```python
from build123d import *

# Parameters (mm, degrees)
SKETCH2_R          = 50
CUT_EXTRUDE1_DEPTH = 10
SKETCH3_R          = 1
CUT_EXTRUDE2_DEPTH = 180
SKETCH4_R          = 1
CUT_EXTRUDE3_DEPTH = 1
SKETCH5_R          = 99.5
CUT_EXTRUDE7_DEPTH = 26


with BuildPart() as part:
    # Sketch1 → Revolve1 (revolve)
    with BuildSketch(Plane.XY):
        Polygon((0, 0), (50, 0), (200, 50), (200, 101), (0, 101), align=None)
        Polygon((49.83772234, 1), (199, 50.72075922), (199, 100), (1, 100), (1, 1), align=None, mode=Mode.SUBTRACT)
    revolve(axis=Axis((0, 101, 0), (1, 0, 0)))

    # Sketch2 → Cut-Extrude1 (cut)
    with BuildSketch(Plane(origin=(200, 0, 0), x_dir=(0, 0, -1), z_dir=(1, 0, 0))):
        with Locations((0, 101)):
            Circle(SKETCH2_R)
    extrude(amount=-CUT_EXTRUDE1_DEPTH, mode=Mode.SUBTRACT)

    # Sketch3 → Cut-Extrude2 (cut)
    with BuildSketch(Plane(origin=(190, 0, 0), x_dir=(0, 0, -1), z_dir=(1, 0, 0))):
        with Locations((0, 101)):
            Circle(SKETCH3_R)
    extrude(amount=-CUT_EXTRUDE2_DEPTH, mode=Mode.SUBTRACT)

    # Sketch4 → Cut-Extrude3 (cut)
    with BuildSketch(Plane(origin=(10, 0, 0), x_dir=(0, 0, -1), z_dir=(1, 0, 0))):
        with Locations((0, 101)):
            Circle(SKETCH4_R)
    extrude(amount=-CUT_EXTRUDE3_DEPTH, mode=Mode.SUBTRACT)

    # Sketch5 → Cut-Extrude7 (cut)
    with BuildSketch(Plane.ZY):
        with Locations((0, 101)):
            Circle(SKETCH5_R)
    extrude(amount=-CUT_EXTRUDE7_DEPTH, mode=Mode.SUBTRACT)


solid = part.part
```
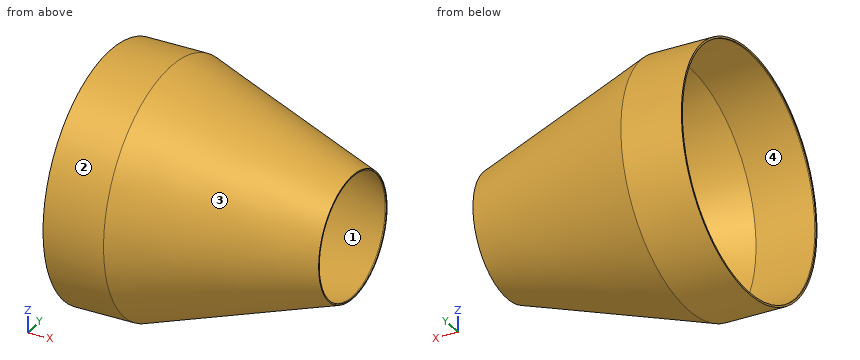
Build history of the part. All positions in model axes, mm. Face numbers are marked on the shaded views. A direction names the side the tool comes from. Give positions to 0.01 mm unless a question says otherwise; leave off trailing zeros. Loops run counter-clockwise (first coordinate to the right, second up) from the corner with the lowest first, then second, coordinate; pieces in that order, holes last.
1) 3-axis set-ups, long thin cutter, end or side, ignore diameter. For the marked faces 3 and 4: which of +Z, -Z, +X, -X, +Y, -Y reach the whole face in a straight line?
Values follow:
face 3: +X
face 4: none
2) Band-saw the part on C-C on x = 33. List the corners of the cut face in (y, z).
Values follow:
outline: circle Ø202 at (101, 0); hole circle Ø200 at (101, 0)
3) Drop flat-ended pins along their axis: P1, Ø4, axis at x = 120.5, y = 161, coming from the -Z side; P2, Ø1.5, axis at x = 159.5, y = 127.5, coming from the -Z side; P3, Ø1.5, axis at x = 165.5, z = 26, coming from the +Y side. Give the stop position or say it passes through.
Values follow:
P1: stops at z = -51.62
P2: stops at z = -59.24
P3: stops at y = 158.27
4) Two-plate mould, pull along Z, no slides. Class the marked faces 1 and 2: released by +Z, released by -Z, zero draft, split by the parting line, or undercut.
Values follow:
face 1: undercut
face 2: split by the parting line
5) Band-saw the part on D-D on x = 84. List the corners of the cut face in (y, z).
Values follow:
outline: circle Ø179.33 at (101, 0); hole circle Ø177.23 at (101, 0)
6) Probe line 1 along Z through (x, y) = (32, 101); line 2 along Y through (x, z) = (0.3, 0); line 3 along Y through (x, z) = (25, 0). List the from-to ranges inside material, lowest first.
Values follow:
line 1: z = -101 to -100, 100 to 101
line 2: y = 0 to 1.5, 200.5 to 202
line 3: y = 0 to 1, 201 to 202
7) Band-saw the part on A-A on y = 101. List the corners of the cut face in (x, z), then the cut area to 3 significant figures.
Values follow:
outline: (0, -101) - (50, -101) - (200, -51) - (200, -50) - (199, -50) - (199, -50.28) - (49.84, -100) - (1, -100) - (1, -99.5) - (0, -99.5) - close; (0, 99.5) - (1, 99.5) - (1, 100) - (49.84, 100) - (199, 50.28) - (199, 50) - (200, 50) - (200, 51) - (50, 101) - (0, 101) - close
area: 417 mm2
8) Band-saw the part on B-B on z = 0. List the corners of the cut face in (x, y).
Values follow:
outline: (0, 0) - (50, 0) - (200, 50) - (200, 51) - (199, 51) - (199, 50.72) - (49.84, 1) - (1, 1) - (1, 1.5) - (0, 1.5) - close; (0, 200.5) - (1, 200.5) - (1, 201) - (49.84, 201) - (199, 151.28) - (199, 151) - (200, 151) - (200, 152) - (50, 202) - (0, 202) - close
